from build123d import *

# Parameters (mm, degrees)
REVOLVE1_ANGLE = 1


with BuildPart() as part:
    # Sketch1 → Revolve1 (revolve)
    with BuildSketch(Plane.XY):
        with BuildLine():
            Line((-6.858, 0), (6.858, 0))
            Line((6.858, 0), (6.858, 8.89))
            Line((6.858, 8.89), (2.848341014, 8.89))
            ThreePointArc((2.848341014, 8.89), (2.598655598, 8.76001488), (2.561932025, 8.480926511))
            Line((2.561932025, 8.480926511), (3.761907297, 5.1849418))
            ThreePointArc((3.761907297, 5.1849418), (3.716002836, 4.83608138), (3.403896102, 4.6736))
            Line((3.403896102, 4.6736), (-3.403896102, 4.6736))
            ThreePointArc((-3.403896102, 4.6736), (-3.716002836, 4.83608138), (-3.761907297, 5.1849418))
            Line((-3.761907297, 5.1849418), (-2.561932025, 8.480926511))
            ThreePointArc((-2.561932025, 8.480926511), (-2.598655598, 8.76001488), (-2.848341014, 8.89))
            Line((-2.848341014, 8.89), (-6.858, 8.89))
            Line((-6.858, 8.89), (-6.858, 0))
        make_face()
    revolve(axis=Axis((-133.858, 15.851032083, 0), (0, -1, 0)), revolution_arc=REVOLVE1_ANGLE)


solid = part.part
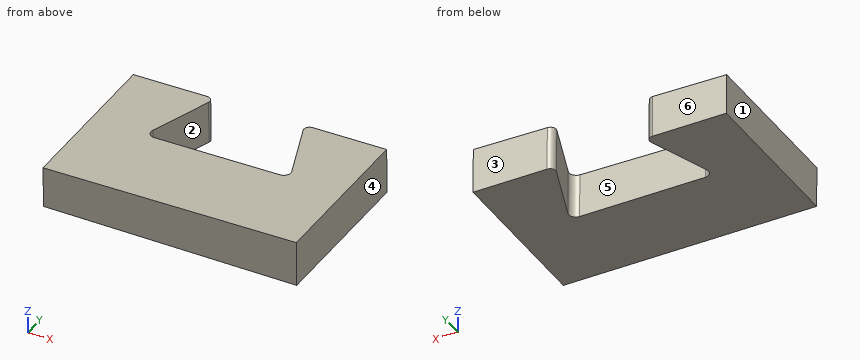
Part model, mm, in its own coordinate system. Face numbers are marked on the shaded views. A direction names the side the tool comes from. Coordinates: 2 decimals unless noted, no trailing zeros. Write each loop counter-clockwise with the first axis right and the second up, starting at its lowest first coordinate (ties: lowest second). Pieces come first, ordered by that corner, then holes. Notation, with made-up numbers: M 18,85 L 52,85 A27 cw 52,108 Z; hole C 47.5,-28.75 d11. An arc over 180 degrees is marked long. Return JSON: item names as keys, results as strings.
1. 3-axis set-ups, long thin cutter, end or side, ignore diameter. For the marked faces 4, 5 and 6: which of +Z, -Z, +X, -X, +Y, -Y reach the whole face in a straight line?
Determined:
{"face 4": "+Z, +X, +Y, -Y", "face 5": "+Z, -Z", "face 6": "+Z, -Z, +X, -X, +Y"}
2. Saw through at A-A, the plane y = 5.75. Write the cut outline in (x, z), then the cut area to 3 significant figures.
Determined:
{"outline": "M -6.88,2.22 A127 cw -6.86,0 L -3.56,0 A130.3 ccw -3.58,2.27 Z; M 3.54,2.4 A137.41 cw 3.56,0 L 6.86,0 A140.72 ccw 6.84,2.46 Z", "area": "15.4 mm²"}
3. Saw through at D-D, the plane y = 8. Write the cut outline in (x, z), then the cut area to 3 significant figures.
Determined:
{"outline": "M -6.88,2.22 A127 cw -6.86,0 L -2.74,0 A131.12 ccw -2.76,2.29 Z; M 2.72,2.38 A136.6 cw 2.74,0 L 6.86,0 A140.72 ccw 6.84,2.46 Z", "area": "19.3 mm²"}
4. Flat gauge pins, fed straight in: pin 1 Ø3 at (x, y) = (4.5, 3.5) entering from +Z; pin 2 Ø1.2 at (x, z) = (1.5, 1) entering from +Y. Where does each tip first touch, or does it go through?
Determined:
{"pin 1": "z = 2.44", "pin 2": "y = 4.67"}
5. Saw through at B-B, the plane y = 2.75. Write the cut outline in (x, z), then the cut area to 3 significant figures.
Determined:
{"outline": "M -6.88,2.22 A127 cw -6.86,0 L 6.86,0 A140.72 ccw 6.84,2.46 Z", "area": "32.0 mm²"}
6. Pull direction Y, two halves, no side cores. Call the marked faces 1, 2 and 3: pulls with the +Y half, pulls with the -Y half, needs draft (parallel to the pull), parting line crosses it, or undercut.
Determined:
{"face 1": "needs draft", "face 2": "undercut", "face 3": "pulls with the +Y half"}
7. Saw through at C-C, the plane x = -6. Write the cut outline in (y, z).
Determined:
{"outline": "M 0,0 L 8.89,0 L 8.89,2.23 L 0,2.23 Z"}
8. Probe L1, parallel to X at y = 5.5, z = 0.7; L2, parallel to X at y = 7.5, z = 1.9; L3, parallel to Y at x = 0.5, z = 2.15. List the from-to ranges inside material, lowest first.
Determined:
{"L1": "-6.86 to -3.65, 3.65 to 6.86", "L2": "-6.87 to -2.93, 2.91 to 6.85", "L3": "0 to 4.67"}
